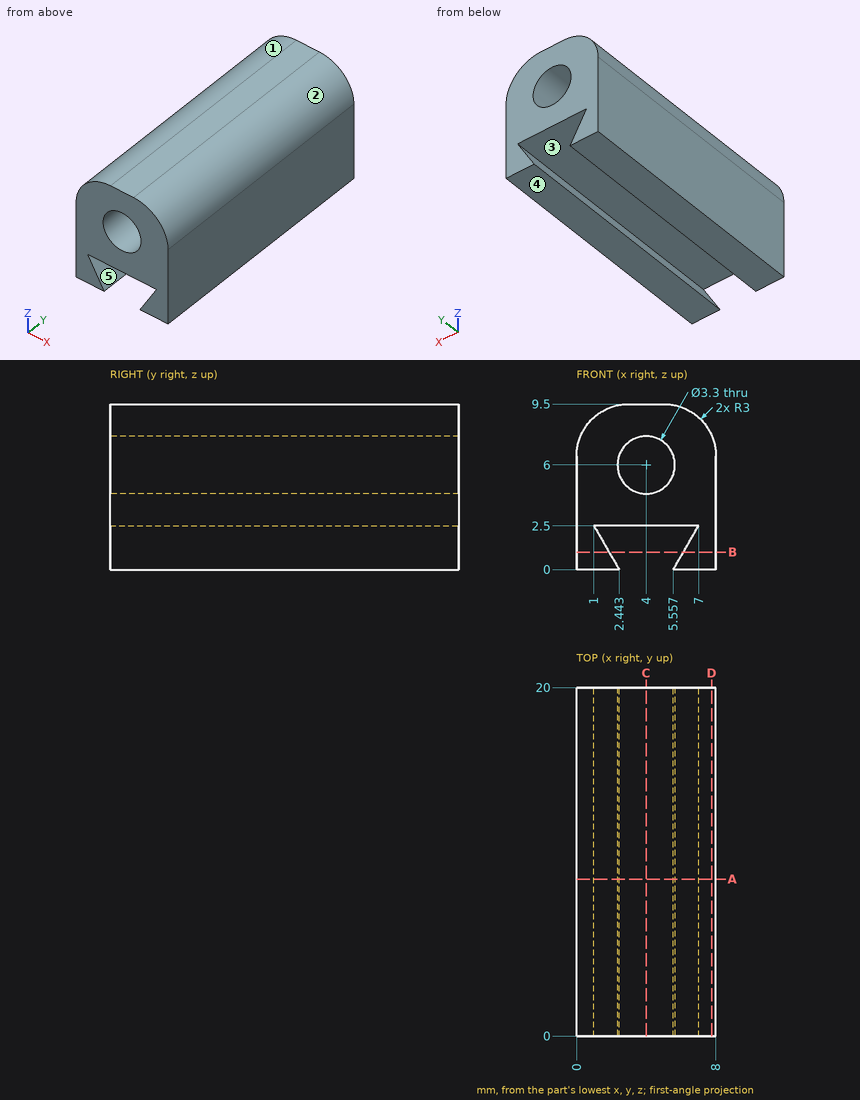
Input: dimensioned drawing with shaded views. Units: mm. Origin: part minimum x, y, z. A direction names the side the tool comes from. Coordinates: 2 decimals unless noted, no trailing zeros. Loops run counter-clockwise (first coordinate to the right, second up) from the corner with the lowest first, then second, coordinate; pieces in that order, holes last. Notation, with made-up numbers: M -1,-40 L 37,-40 A12 cw 37,-23 Z; hole C -19,-32.75 d5. An arc over 180 degrees is marked long. One line per item, written item: value. Start each with the question number.
1) Cut plane A-A (y = 9). Return loops of the section in (x, z), then the cut area to 3 significant figures.
2) Pin query (flat end, axial travel): P1, Ø2, axis at x = 4.5, y = 8.5, coming from the -Z side; P2, Ø1, axis at y = 9, z = 2.5, coming from the -X side. Return the tip coordinate at first contact, or that it passes through.
3) Cut plane C-C (x = 4). Return loops of the section in (y, z).
4) Draft query along X for the marked faces 1, 2 and 3. Return one class per face: released by +X, released by -X, zero draft, split by the parting line, or undercut.
5) Reachability of the marked faces 4 and 5 from +Z, -Z, +X, -X, +Y, -Y: full face, straight path, thin tool, end or side. Return the list, or none.
6) Cut plane B-B (z = 1). Return loops of the section in (x, y).
7) Material intervals for L1, parallel to Z at x = 4, y = 9; L2, parallel to X at y = 9.75, z = 6; L3, parallel to Z at x = 2.5, y = 4.5 (1 decimal), sorted ascending. Write a range as from..to.
8) Cut plane D-D (x = 7.75). Return loops of the section in (y, z), then the cut area to 3 significant figures.
Evaluation:
1. outline: M 0,0 L 2.44,0 L 1,2.5 L 7,2.5 L 5.56,0 L 8,0 L 8,6.5 A3 ccw 5,9.5 L 3,9.5 A3 ccw 0,6.5 Z; hole C 4,6 d3.3
1. area: 52.2 mm^2
2. P1: z = 2.5
2. P2: x = 0
3. outline: M 0,2.5 L 20,2.5 L 20,4.35 L 0,4.35 Z; M 0,7.65 L 20,7.65 L 20,9.5 L 0,9.5 Z
4. face 1: released by -X
4. face 2: released by +X
4. face 3: undercut
5. face 4: -Z, +X, -X, +Y, -Y
5. face 5: +Y, -Y
6. outline: M 0,0 L 1.87,0 L 1.87,20 L 0,20 Z; M 6.13,0 L 8,0 L 8,20 L 6.13,20 Z
7. L1: 2.5..4.35, 7.65..9.5
7. L2: 0..2.35, 5.65..8
7. L3: 2.5..5.3, 6.7..9.5
8. outline: M 0,0 L 20,0 L 20,7.7 L 0,7.7 Z
8. area: 154 mm^2
